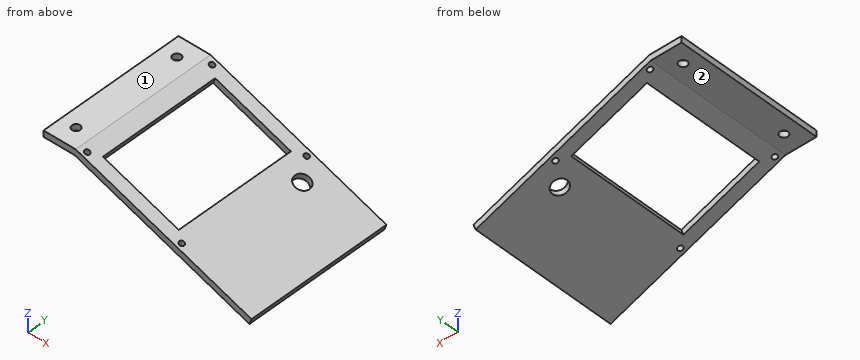
```python
from build123d import *

# Parameters (mm, degrees)
SKETCH1_W           = 95
SKETCH1_H           = 20
SKETCH1_R           = 2.65
BOSS_EXTRUDE1_DEPTH = 4
BOSS_EXTRUDE2_DEPTH = 95
SKETCH3_R           = 1.65
SKETCH3_R_2         = 5
SKETCH3_W           = 79
SKETCH3_H           = 52
CUT_EXTRUDE1_DEPTH  = 140.048139578


with BuildPart() as part:
    # Sketch1 → Boss-Extrude1 (new body)
    with BuildSketch(Plane(origin=(0, 0, 0), x_dir=(0, 1, 0), z_dir=(0, 0, 1))):
        Rectangle(SKETCH1_W, SKETCH1_H)
        with Locations(Location((35.5, 0, 0), (0, 0, 270))):
            Circle(SKETCH1_R, mode=Mode.SUBTRACT)
        with Locations(Location((-35.5, 0, 0), (0, 0, 270))):
            Circle(SKETCH1_R, mode=Mode.SUBTRACT)
    extrude(amount=BOSS_EXTRUDE1_DEPTH)

    # Sketch2 → Boss-Extrude2 (add)
    with BuildSketch(Plane.XZ.offset(47.5)):
        Polygon((10, 0), (122.763114494, -41.042417199), (124.131195068, -37.283646716), (10.705307923, 4), (10, 4), align=None)
    extrude(amount=-BOSS_EXTRUDE2_DEPTH)

    # Sketch3 → Cut-Extrude1 (cut, through all)
    with BuildSketch(Plane(origin=(1.169777784, 0, 3.213938048), x_dir=(0, -1, 0), z_dir=(-0.34202014332566977, 0, -0.9396926207859081))):
        with Locations(Location((43.95, -13.168790985, 0), (0, 0, 90))):
            Circle(SKETCH3_R)
        with Locations(Location((43.95, -78.068790985, 0), (0, 0, 90))):
            Circle(SKETCH3_R)
        with Locations(Location((-43.95, -78.068790985, 0), (0, 0, 90))):
            Circle(SKETCH3_R)
        with Locations(Location((-43.95, -13.168790985, 0), (0, 0, 90))):
            Circle(SKETCH3_R)
        with Locations(Location((-31.1, -87.618790985, 0), (0, 0, 90))):
            Circle(SKETCH3_R_2)
        with Locations((0, -45.618790985)):
            Rectangle(SKETCH3_W, SKETCH3_H)
    extrude(amount=-CUT_EXTRUDE1_DEPTH, mode=Mode.SUBTRACT)


solid = part.part
```
Source: CAD feature listing. Evaluate the final solid. Frame: model axes, mm. Face numbers are marked on the shaded views. A direction names the side the tool comes from. Round coordinates to 2 decimals unless told otherwise and drop trailing zeros. Loops run counter-clockwise (first coordinate to the right, second up) from the corner with the lowest first, then second, coordinate; pieces in that order, holes last.
1. Ray query, L1, parallel to Y at x = 0, z = 1.65; L2, parallel to Y at x = 55.5, z = -13; L3, parallel to Z at x = 83.5, y = -30.5. Return the intervals inside material, ascending.
2. Section query D-D on x = 42.5. Output: boundary loops of the cut face in (y, z), and give its area (3 significant figures).
3. Section query C-C on z = -11.5. Output: boundary loops of the cut face in (x, y), and give its area (3 significant figures).
4. Access query for the marked faces 1 and 2. Directions: +Z, -Z, +X, -X, +Y, -Y. A direction counts if a zero-diameter tool reaches every point of the face in a straight line with its end or side. Return the directions, or none.
5. Section query B-B on x = 0. Output: boundary loops of the cut face in (y, z).
6. Contact query for flat-ended pins moving along their axis: pin 1 (7 mm diameter, centred on x = 0, y = 35.5, fed in from -Z); pin 2 (3 mm diameter, centred on y = -31.5, z = -18, fed in from -X); pin 3 (4 mm diameter, centred on x = 92.5, y = -1.5, fed in from -Z). Output: stop coordinate, or through.
7. Section query A-A on y = 7. Output: boundary loops of the cut face in (x, z), and give its area (3 significant figures).
Answers below:
1. L1: y = -47.5 to -38.15, -32.85 to 32.85, 38.15 to 47.5
1. L2: y = -47.5 to -39.5, 39.5 to 47.5
1. L3: z = -26.75 to -22.5
2. outline: (-47.5, -11.83) - (-39.5, -11.83) - (-39.5, -7.57) - (-47.5, -7.57) - close; (39.5, -11.83) - (47.5, -11.83) - (47.5, -7.57) - (39.5, -7.57) - close
2. area: 68.1 mm2
3. outline: (41.6, -47.5) - (53.29, -47.5) - (53.29, -39.5) - (41.6, -39.5) - close; (41.6, 39.5) - (53.29, 39.5) - (53.29, 47.5) - (41.6, 47.5) - close
3. area: 187 mm2
4. face 1: +Z, +X, -X, +Y, -Y
4. face 2: -Z, -X, +Y, -Y
5. outline: (-47.5, 0) - (-38.15, 0) - (-38.15, 4) - (-47.5, 4) - close; (-32.85, 0) - (32.85, 0) - (32.85, 4) - (-32.85, 4) - close; (38.15, 0) - (47.5, 0) - (47.5, 4) - (38.15, 4) - close
6. pin 1: stops at z = 0
6. pin 2: stops at x = 69.12
6. pin 3: stops at z = -30.76
7. outline: (-10, 0) - (10, 0) - (19.61, -3.5) - (20.97, 0.26) - (10.71, 4) - (-10, 4) - close; (68.47, -21.28) - (122.76, -41.04) - (124.13, -37.28) - (69.84, -17.52) - close
7. area: 355 mm2
